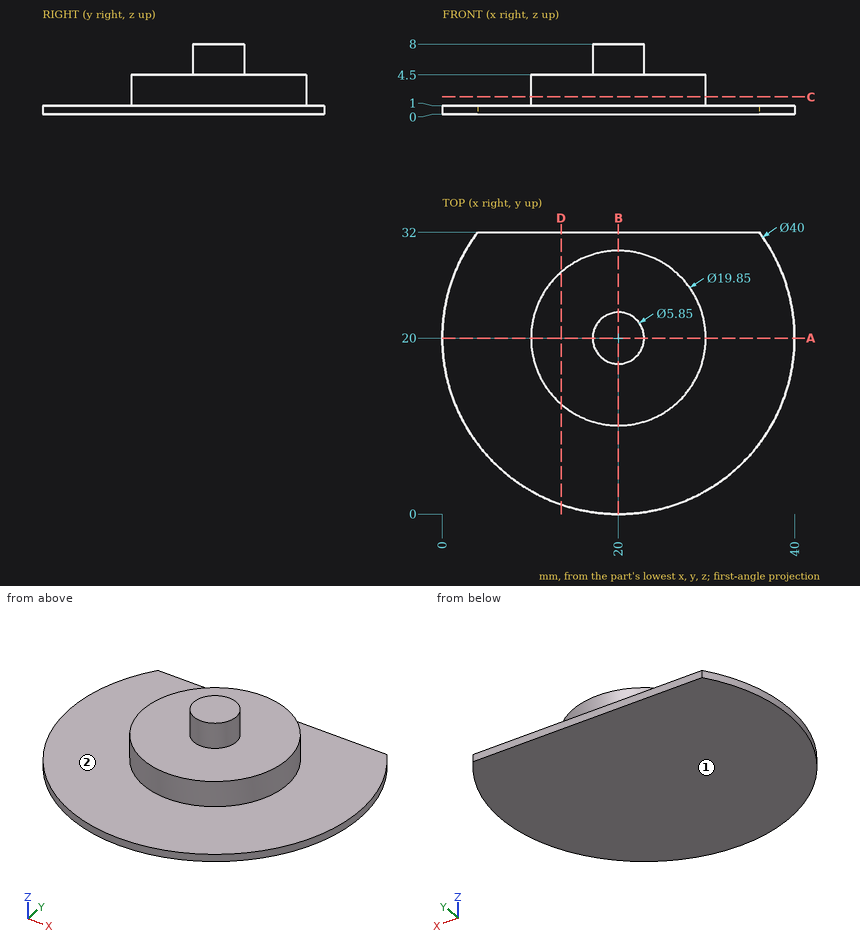
Design review of the part shown in the three views and the two pictorial views. Dimensions are in mm from the part's minimum x, y and z. A direction names the side the tool comes from. Coordinates: 2 decimals unless noted, no trailing zeros. Order: outer loops, then holes, each group sorted by start corner. A loop starts at its lowest first (then second) coordinate and runs counter-clockwise, first axis right, second up.
Item 1: For pin 1 Ø2 at (x, z) = (27, 2.5) entering from -Y; pin 2 Ø10 at (x, y) = (28, 24) entering from +Z, all flat-tipped, find the tip position at first contact; note any pin that passes through.
Item 2: For line 1 (Z direction, x = 16.5, y = 15.5); line 2 (Z direction, x = 9.5, y = 7); line 3 (Y direction, x = 20, z = 7.5) (3 decimals), list the stretches that pass through material, from the lowest coordinate up.
Item 3: Take a section at A-A, the plane y = 20. Write out the cut boundary in (x, z) (3 decimals), then the cut area to 3 significant figures.
Item 4: Take a section at C-C, the plane z = 2. Write out the cut boundary in (x, y) (3 decimals).
Item 5: For the marked faces 1 and 2, list the 3-axis set-ups (+Z, -Z, +X, -X, +Y, -Y) from which the entire face can be reached by the end or side of a thin tool; tool diameter is ignored.
Item 6: Take a section at D-D, the plane x = 13.5. Write out the cut boundary in (y, z).
Item 7: Take a section at B-B, the plane x = 20. Write out the cut boundary in (y, z) (3 decimals), then the cut area to 3 significant figures.
The answers:
1. pin 1: stops at y = 12.09
1. pin 2: stops at z = 4.5
2. line 1: z = 0 to 4.5
2. line 2: z = 0 to 1
2. line 3: y = 17.075 to 22.925
3. outline: (0, 0) - (40, 0) - (40, 1) - (29.925, 1) - (29.925, 4.5) - (22.925, 4.5) - (22.925, 8) - (17.075, 8) - (17.075, 4.5) - (10.075, 4.5) - (10.075, 1) - (0, 1) - close
3. area: 130 mm2
4. outline: circle Ø19.85 at (20, 20)
5. face 1: -Z, +X, -X, +Y, -Y
5. face 2: +Z
6. outline: (1.09, 0) - (32, 0) - (32, 1) - (27.5, 1) - (27.5, 4.5) - (12.5, 4.5) - (12.5, 1) - (1.09, 1) - close
7. outline: (0, 0) - (32, 0) - (32, 1) - (29.925, 1) - (29.925, 4.5) - (22.925, 4.5) - (22.925, 8) - (17.075, 8) - (17.075, 4.5) - (10.075, 4.5) - (10.075, 1) - (0, 1) - close
7. area: 122 mm2
